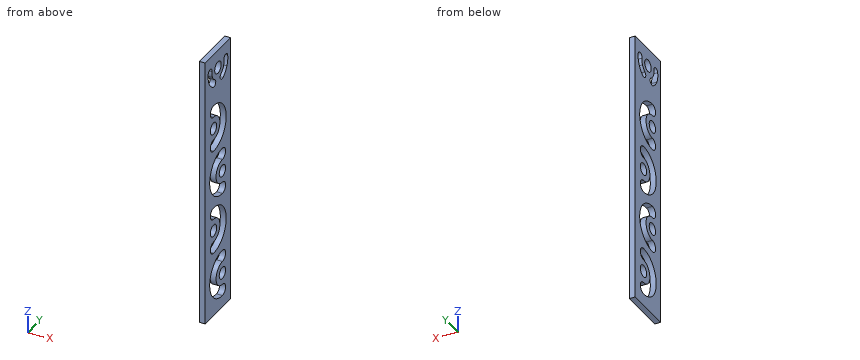
```python
from build123d import *

# Parameters (mm, degrees)
F0_W      = 63.5
F0_H      = 63.5
F0_W_2    = 50.8
F0_H_2    = 50.8
F1_DEPTH  = 165.1
F3_R      = 6.477
F4_DEPTH  = 25.4
F6_DEPTH  = 25.4
F7_R      = 6.35
F8_DEPTH  = 63.501
F9_W      = 93.0855199695
F9_H      = 380.0157606602
F9_W_2    = 50.8
F9_H_2    = 292.1
F10_DEPTH = 38.1
F11_W     = 93.9574092627
F11_H     = 381.9095790386
F12_DEPTH = 91.44


# Not quite as in the source:
# - ends of sketch curves that miss each other by under 0.0002 mm in the source are joined


with BuildPart() as f1:
    # F0 (on Top) → F1 (new body, symmetric)
    with BuildSketch(Plane.XY):
        Rectangle(F0_W, F0_H)
        Rectangle(F0_W_2, F0_H_2, mode=Mode.SUBTRACT)
    extrude(amount=F1_DEPTH, both=True)

    # F3 (on face) → F4 (cut)
    with BuildSketch(Plane.YZ.offset(31.75)):
        with Locations((0, 146.05)):
            Circle(F3_R)
        with BuildLine():
            ThreePointArc((10.1385245046, 129.1766616857), (14.6288058895, 132.8781640138), (17.8406687878, 137.7307595176))
            ThreePointArc((17.8406687878, 137.7307595176), (19.4934269332, 143.3103775076), (19.4426449846, 149.1294124443))
            ThreePointArc((19.4426449846, 149.1294124443), (15.0835370951, 152.2964897102), (11.9164598293, 147.9373818207))
            ThreePointArc((11.9164598293, 147.9373818207), (11.9475842494, 144.3708765369), (10.9346034506, 140.9511106721))
            ThreePointArc((10.9346034506, 140.9511106721), (8.9660423194, 137.9769392343), (6.2139343738, 135.708276517))
            ThreePointArc((6.2139343738, 135.708276517), (4.9104220235, 130.4801740359), (10.1385245046, 129.1766616857))
        make_face()
        with BuildLine():
            ThreePointArc((-10.1385245046, 129.1766616857), (-4.9104220235, 130.4801740359), (-6.2139343738, 135.708276517))
            ThreePointArc((-6.2139343738, 135.708276517), (-8.9660423194, 137.9769392343), (-10.9346034506, 140.9511106721))
            ThreePointArc((-10.9346034506, 140.9511106721), (-11.9475842494, 144.3708765369), (-11.9164598293, 147.9373818207))
            ThreePointArc((-11.9164598293, 147.9373818207), (-15.0835370951, 152.2964897102), (-19.4426449846, 149.1294124443))
            ThreePointArc((-19.4426449846, 149.1294124443), (-19.4934269332, 143.3103775076), (-17.8406687878, 137.7307595176))
            ThreePointArc((-17.8406687878, 137.7307595176), (-14.6288058895, 132.8781640138), (-10.1385245046, 129.1766616857))
        make_face()
    extrude(amount=-F4_DEPTH, mode=Mode.SUBTRACT)

    # F5 (on face) → F6 (cut)
    with BuildSketch(Plane(origin=(-31.75, 0, 0), x_dir=(0, -1, 0), z_dir=(-1, 0, 0))):
        with BuildLine():
            ThreePointArc((-3.1401119103, 140.3850881569), (3.2873259769, 140.4692279278), (6.477, 146.05))
            ThreePointArc((6.477, 146.05), (-3.2873259769, 151.6307720722), (-3.1401119103, 140.3850881569))
        make_face()
        with BuildLine():
            ThreePointArc((-5.7913527214, 132.1654121492), (-6.0549491708, 133.1322727306), (-6.7727903948, 133.8315626913))
            ThreePointArc((-6.7727903948, 133.8315626913), (-9.3377562721, 131.1985515677), (-5.7913527214, 132.1654121492))
        make_face()
        with BuildLine():
            ThreePointArc((3.1226517792, 134.3961049058), (0.4285749428, 129.7298269458), (5.0948529028, 127.0357501095))
            ThreePointArc((5.0948529028, 127.0357501095), (17.8406687878, 137.7307595176), (17.8406687878, 154.3692404824))
            ThreePointArc((17.8406687878, 154.3692404824), (12.777460542, 156.2120975737), (10.9346034506, 151.1488893279))
            ThreePointArc((10.9346034506, 151.1488893279), (10.9346034506, 140.9511106721), (3.1226517792, 134.3961049058))
        make_face()
    extrude(amount=-F6_DEPTH, mode=Mode.SUBTRACT)

    # F7 (on face) → F8 (cut, through all)
    with BuildSketch(Plane.YZ.offset(31.75)):
        with BuildLine():
            ThreePointArc((-8.89, 107.949999693), (-15.239999693, 101.6), (-8.89, 95.250000307))
            ThreePointArc((-8.89, 95.250000307), (3.81, 82.55), (-8.89, 69.85))
            ThreePointArc((-8.89, 69.85), (-15.239999693, 63.5), (-8.89, 57.150000307))
            ThreePointArc((-8.89, 57.150000307), (16.509999693, 82.55), (-8.89, 107.949999693))
        make_face()
        with BuildLine():
            ThreePointArc((8.89, 3.07e-07), (15.239999693, 6.35), (8.89, 12.699999693))
            ThreePointArc((8.89, 12.699999693), (-3.81, 25.4), (8.89, 38.1))
            ThreePointArc((8.89, 38.1), (15.24, 44.45), (8.89, 50.8))
            ThreePointArc((8.89, 50.8), (-16.509999693, 25.4), (8.89, 3.07e-07))
        make_face()
        with BuildLine():
            ThreePointArc((-8.89, -6.350000307), (-15.239999693, -12.7), (-8.89, -19.049999693))
            ThreePointArc((-8.89, -19.049999693), (3.81, -31.75), (-8.89, -44.45))
            ThreePointArc((-8.89, -44.45), (-15.239999693, -50.8), (-8.89, -57.149999693))
            ThreePointArc((-8.89, -57.149999693), (16.509999693, -31.75), (-8.89, -6.350000307))
        make_face()
        with BuildLine():
            ThreePointArc((8.89, -114.299999693), (15.239999693, -107.95), (8.89, -101.600000307))
            ThreePointArc((8.89, -101.600000307), (-3.81, -88.9), (8.89, -76.2))
            ThreePointArc((8.89, -76.2), (15.24, -69.85), (8.89, -63.5))
            ThreePointArc((8.89, -63.5), (-16.509999693, -88.9), (8.89, -114.299999693))
        make_face()
        with Locations((-8.89, 82.55)):
            Circle(F7_R)
        with Locations((8.89, 25.4)):
            Circle(F7_R)
        with Locations((8.89, -88.9)):
            Circle(F7_R)
        with Locations((-8.89, -31.75)):
            Circle(F7_R)
    extrude(amount=-F8_DEPTH, mode=Mode.SUBTRACT)

    # F9 (on face) → F10 (cut, symmetric)
    with BuildSketch(Plane(origin=(25.4, 0, 0), x_dir=(0, -1, 0), z_dir=(-1, 0, 0))):
        Rectangle(F9_W, F9_H)
        with Locations((0, 19.05)):
            Rectangle(F9_W_2, F9_H_2, mode=Mode.SUBTRACT)
    extrude(amount=F10_DEPTH, both=True, mode=Mode.SUBTRACT)

    # F11 (on face) → F12 (cut)
    with BuildSketch(Plane(origin=(25.4, 0, 0), x_dir=(0, -1, 0), z_dir=(-1, 0, 0))):
        Rectangle(F11_W, F11_H)
    extrude(amount=F12_DEPTH, mode=Mode.SUBTRACT)


solid = f1.part
```
Model file for the job. Use its own axes, mm. Give positions to 0.01 mm unless a question says otherwise; leave off trailing zeros. Write each loop counter-clockwise with the first axis right and the second up, starting at its lowest first coordinate (ties: lowest second). Pieces come first, ordered by that corner, then holes. Notation, with made-up numbers: (72, 73.25) - (112, 73.25) arc R12 cw to (112, 92.25) - close; hole circle Ø6 at (-12.75, 42.5). An arc over 180 degrees is marked (long way). One line per question, with ' | ' between items. Start each with the question number.
(1) Pin check, flat tip, straight feed: P1, Ø7.5, axis at y = -8.89, z = 82.55, coming from the +X side. Stop position of the tip, or through.
(2) Slice it at C-C on y = 0. Give the number of separate pieces and of enclosed holes in the cut face, plus the area to 3 significant figures.
(3) Wall check: line 1 along Y through (x, z) = (25.75, -89); line 2 along Y through (x, z) = (28, 28); line 3 along Y through (x, z) = (26.25, 94). Give the ranges that are in metal, low to high. Write a range as from..to.
(4) Slice it at A-A on z = 82.55. Write the cut outline in (x, y), plus the area to 3 significant figures.
(5) Slice it at B-B on z = -22. Write the cut outline in (x, y).
Results below:
1) P1: through
2) separate pieces: 10 | enclosed holes: 0 | area: 1,020 mm^2
3) line 1: -25.4..-16.51, -3.81..2.54, 15.24..25.4 | line 2: -25.4..-16.38, -3.54..3.1, 14.68..25.4 | line 3: -25.4..-3.4, 13.78..25.4
4) outline: (25.4, -25.4) - (31.75, -25.4) - (31.75, -15.24) - (25.4, -15.24) - close; (25.4, -2.54) - (31.75, -2.54) - (31.75, 3.81) - (25.4, 3.81) - close; (25.4, 16.51) - (31.75, 16.51) - (31.75, 25.4) - (25.4, 25.4) - close | area: 161 mm^2
5) outline: (25.4, -25.4) - (31.75, -25.4) - (31.75, -0.75) - (25.4, -0.75) - close; (25.4, 14.56) - (31.75, 14.56) - (31.75, 25.4) - (25.4, 25.4) - close
